Source: CAD feature listing. Evaluate the final solid. Frame: model axes, mm. A direction names the side the tool comes from. Give positions to 0.01 mm unless a question says otherwise; leave off trailing zeros. Loops run counter-clockwise (first coordinate to the right, second up) from the corner with the lowest first, then second, coordinate; pieces in that order, holes last. Notation, with made-up numbers: M 41.5,20.25 L 99.5,20.25 A5 cw 99.5,25.25 Z; hole C 1,88.25 d1. An arc over 180 degrees is marked long. Answer in a Markdown table with one row per item.
```python
from build123d import *

# Parameters (mm, degrees)
SKETCH1_W           = 9.53
SKETCH1_H           = 9.53
BASIC_SHAPE_DEPTH   = 4.83
SKETCH2_R           = 0.25
PINS_DEPTH          = 5
SKETCH3_R           = 2
ADJUSTER_DEPTH      = 0.1
ADJUSTER_SLOT_DEPTH = 1


with BuildPart() as part:
    # Sketch1 → Basic Shape (new body)
    with BuildSketch(Plane(origin=(0, 0, 0), x_dir=(1, 0, 0), z_dir=(0, 0, -1))):
        with Locations((4.765, 4.765)):
            Rectangle(SKETCH1_W, SKETCH1_H)
    extrude(amount=BASIC_SHAPE_DEPTH)

    # Sketch2 → Pins (add)
    with BuildSketch(Plane.XY.offset(-4.83)):
        with Locations((4.8, -7.305)):
            Circle(SKETCH2_R)
        with Locations((4.8, -2.225)):
            Circle(SKETCH2_R)
        with Locations((7.34, -4.765)):
            Circle(SKETCH2_R)
    extrude(amount=-PINS_DEPTH)

    # Sketch3 → Adjuster (cut)
    with BuildSketch(Plane(origin=(0, 0, 0), x_dir=(-1, 0, 0), z_dir=(0, 0, -1))):
        with Locations((-4.765, -4.765)):
            Circle(SKETCH3_R)
    extrude(amount=ADJUSTER_DEPTH, mode=Mode.SUBTRACT)

    # Sketch4 → Adjuster Slot (cut)
    with BuildSketch(Plane(origin=(0, 0, -0.1), x_dir=(-1, 0, 0), z_dir=(0, 0, 1))):
        with BuildLine():
            Line((-6.487859784, 3.749246997), (-3.749246997, 6.487859784))
            ThreePointArc((-3.749246997, 6.487859784), (-3.350786438, 6.179213562), (-3.042140216, 5.780753003))
            Line((-3.042140216, 5.780753003), (-5.780753003, 3.042140216))
            ThreePointArc((-5.780753003, 3.042140216), (-6.179213562, 3.350786438), (-6.487859784, 3.749246997))
        make_face()
    extrude(amount=-ADJUSTER_SLOT_DEPTH, mode=Mode.SUBTRACT)


solid = part.part
```
1) Section D-D, the plane x = 4. Return loops of the section in (y, z).
Reply:
| item | result |
|---|---|
| outline | M -9.53,-4.83 L 0,-4.83 L 0,0 L -2.92,0 L -2.92,-0.1 L -4.82,-0.1 L -4.82,-1.1 L -6.24,-1.1 L -6.24,-0.1 L -6.61,-0.1 L -6.61,0 L -9.53,0 Z |
2) Material intervals for L1, parallel to Z at x = 8, y = -1.75; L2, parallel to Y at x = 3.5, z = -0.5; L3, parallel to Z at x = 4, y = -5, sorted ascending.
Reply:
| item | result |
|---|---|
| L1 | z = -4.83 to 0 |
| L2 | y = -9.53 to -6.31, -5.32 to 0 |
| L3 | z = -4.83 to -1.1 |
3) Section A-A, the plane x = 7.34. Return loops of the section in (y, z) (3 decimals).
Reply:
| item | result |
|---|---|
| outline | M -9.53,-4.83 L -5.015,-4.83 L -5.015,-9.83 L -4.515,-9.83 L -4.515,-4.83 L 0,-4.83 L 0,0 L -9.53,0 Z |
4) Section C-C, the plane z = -7.25. Return loops of the section in (x, y) (3 decimals), then the cut area to 3 significant figures.
Reply:
| item | result |
|---|---|
| outline | C 4.8,-7.305 d0.5; C 4.8,-2.225 d0.5; C 7.34,-4.765 d0.5 |
| area | 0.589 mm² |
5) Set-up query: faces 1 (the flat face through (0, -5, -2)), 2 (the flat face through (4, -4, -0.1)). Return all of +Z, -Z, +X, -X, +Y, -Y with unobstructed straight access to the full face (end or side cutting, diameter ignored); none if empty.
Reply:
| item | result |
|---|---|
| face 1 | +Z, -Z, -X, +Y, -Y |
| face 2 | +Z |
6) Pull-direction query (Y, two-part tool) for faces 3 (the flat face through (5.138, -5.099, -0.593)), 4 (the flat face through (5, 0, -2)), 5 (the flat face through (5, -9.53, -2)); classes: released by +Y, released by -Y, zero draft, split by the parting line, or undercut.
Reply:
| item | result |
|---|---|
| face 3 | undercut |
| face 4 | released by +Y |
| face 5 | released by -Y |
7) Section B-B, the plane y = -4.25. Return loops of the section in (x, z), then the cut area to 3 significant figures.
Reply:
| item | result |
|---|---|
| outline | M 0,-4.83 L 9.53,-4.83 L 9.53,0 L 6.7,0 L 6.7,-0.1 L 5.99,-0.1 L 5.99,-1.1 L 4.57,-1.1 L 4.57,-0.1 L 2.83,-0.1 L 2.83,0 L 0,0 Z |
| area | 44.2 mm² |
8) Pin query (flat end, axial travel): pin 1 Ø2 at (x, y) = (6.5, -7.5) entering from -Z; pin 2 Ø1.7 at (x, y) = (5.5, -5) entering from +Z. Return the tip coordinate at first contact, or that it passes through.
Reply:
| item | result |
|---|---|
| pin 1 | stops at z = -4.83 |
| pin 2 | stops at z = -0.1 |
